Verification items for this drawing (mm, ordinates from the low corner). A direction names the side the tool comes from. Give positions to 0.01 mm unless a question says otherwise; leave off trailing zeros. Loops run counter-clockwise (first coordinate to the right, second up) from the corner with the lowest first, then second, coordinate; pieces in that order, holes last. Notation, with made-up numbers: (-6, 12) -> (27, 12) arc R29 ccw to (27, 35) -> close; hole circle Ø5 at (-36.5, -9). An arc over 180 degrees is marked (long way). Answer in a Markdown table with one row per item. Add a question column.
Q1. Section check C-C on y = 0.6. Enter the section's corners in (x, z).
Q2. Section check B-B on x = 6. Enter the section's corners in (y, z).
Q3. Material ranges on probe 1 along X at (y, z) = (2.6, 16.75); probe 2 along Z at (x, y) = (8, 3.6); probe 3 along X at (y, z) = (2.2, 9.75), recorded low to high.
Q4. Section check A-A on z = 16.75. Enter the section's corners in (x, y), and give its area (3 significant figures).
Q5. Release check for a two-part mould opening along X. For the marked faces 4, 5, 6 and 7 record: pulls with the +X half, pulls with the -X half, needs draft (parallel to the pull), parting line crosses it, or undercut.
Q6. Section check D-D on z = 10.25. Enter the section's corners in (x, y).
Q7. Gauge pin test, flat ends, axial feed: P1, Ø0.9, axis at y = 1, z = 9.5, coming from the +X side; P2, Ø1.5, axis at x = 5, z = 16.75, coming from the +Y side. Record the tip position at first contact, or that the pin passes through.
Q8. Set-up check for the marked faces 1, 2 and 3: record each of +Z, -Z, +X, -X, +Y, -Y from which the full face is reachable in a straight line by a thin tool's end or side.
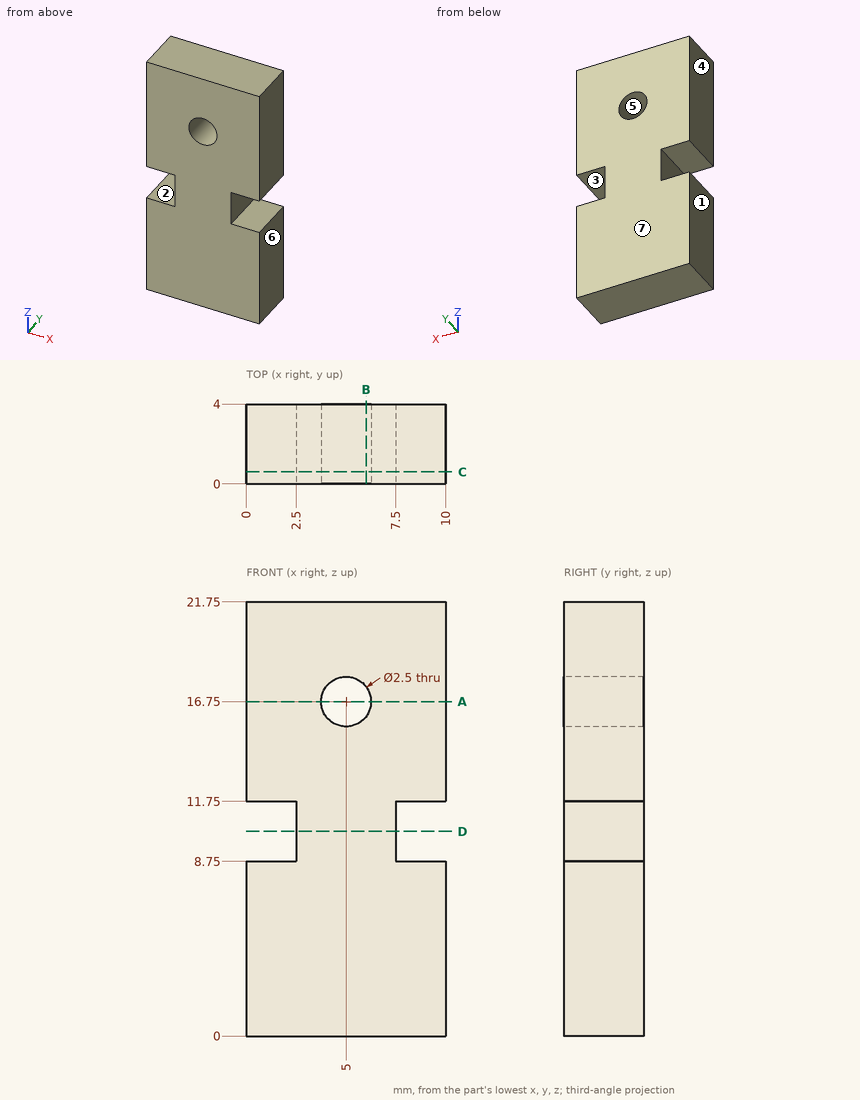
Taken from the geometry:
| question | item | result |
|---|---|---|
| 1 | outline | (0, 0) -> (10, 0) -> (10, 8.75) -> (7.5, 8.75) -> (7.5, 11.75) -> (10, 11.75) -> (10, 21.75) -> (0, 21.75) -> (0, 11.75) -> (2.5, 11.75) -> (2.5, 8.75) -> (0, 8.75) -> close; hole circle Ø2.5 at (5, 16.75) |
| 2 | outline | (0, 0) -> (4, 0) -> (4, 16) -> (0, 16) -> close; (0, 17.5) -> (4, 17.5) -> (4, 21.75) -> (0, 21.75) -> close |
| 3 | probe 1 | x = 0 to 3.75, 6.25 to 10 |
| 3 | probe 2 | z = 0 to 8.75, 11.75 to 21.75 |
| 3 | probe 3 | x = 2.5 to 7.5 |
| 4 | outline | (0, 0) -> (3.75, 0) -> (3.75, 4) -> (0, 4) -> close; (6.25, 0) -> (10, 0) -> (10, 4) -> (6.25, 4) -> close |
| 4 | area | 30.0 mm² |
| 5 | face 4 | pulls with the -X half |
| 5 | face 5 | undercut |
| 5 | face 6 | pulls with the +X half |
| 5 | face 7 | needs draft |
| 6 | outline | (2.5, 0) -> (7.5, 0) -> (7.5, 4) -> (2.5, 4) -> close |
| 7 | P1 | stops at x = 7.5 |
| 7 | P2 | passes through |
| 8 | face 1 | +Z, -Z, -X, +Y, -Y |
| 8 | face 2 | -X, +Y, -Y |
| 8 | face 3 | +X, +Y, -Y |
